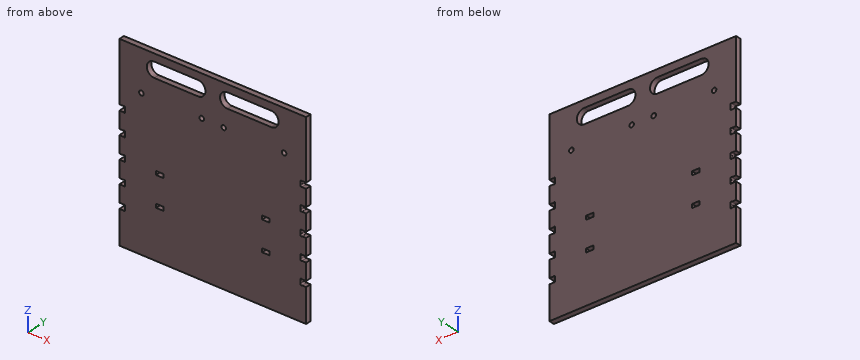
```python
from build123d import *

# Parameters (mm, degrees)
BOSS_EXTRUDE1_DEPTH     = 19.05
SKETCH2_R               = 7.9375
CUT_EXTRUDE1_DEPTH      = 836.260375572
SKETCH3_W               = 25.4
SKETCH3_H               = 12.7
CUT_EXTRUDE2_DEPTH      = 836.260375572
SKETCH4_W               = 444.5
SKETCH4_H               = 114.3
BOSS_EXTRUDE2_DEPTH     = 19.05
CUT_EXTRUDE3_DEPTH      = 836.260375572
CUT_EXTRUDE3_DEPTH_BACK = 836.260375572


with BuildPart() as part:
    # Sketch1 → Boss-Extrude1 (new body)
    with BuildSketch(Plane(origin=(0, 0, 0), x_dir=(1, 0, 0), z_dir=(0, 1, 0))):
        with BuildLine():
            Line((0, 88.9), (0, -114.3))
            Line((0, -114.3), (101.6, -114.3))
            Line((101.6, -114.3), (101.6, 0))
            Line((101.6, 0), (546.1, 0))
            Line((546.1, 0), (546.1, -114.3))
            Line((546.1, -114.3), (647.7, -114.3))
            Line((647.7, -114.3), (647.7, 88.9))
            Line((647.7, 88.9), (633.140128061, 88.9))
            ThreePointArc((633.140128061, 88.9), (628.65, 88.9), (628.65, 93.390128061))
            Line((628.65, 93.390128061), (628.65, 103.459871939))
            ThreePointArc((628.65, 103.459871939), (628.65, 107.95), (633.140128061, 107.95))
            Line((633.140128061, 107.95), (647.7, 107.95))
            Line((647.7, 107.95), (647.7, 165.1))
            Line((647.7, 165.1), (633.140128061, 165.1))
            ThreePointArc((633.140128061, 165.1), (628.65, 165.1), (628.65, 169.590128061))
            Line((628.65, 169.590128061), (628.65, 179.659871939))
            ThreePointArc((628.65, 179.659871939), (628.65, 184.15), (633.140128061, 184.15))
            Line((633.140128061, 184.15), (647.7, 184.15))
            Line((647.7, 184.15), (647.7, 241.3))
            Line((647.7, 241.3), (633.140128061, 241.3))
            ThreePointArc((633.140128061, 241.3), (628.65, 241.3), (628.65, 245.790128061))
            Line((628.65, 245.790128061), (628.65, 255.859871939))
            ThreePointArc((628.65, 255.859871939), (628.65, 260.35), (633.140128061, 260.35))
            Line((633.140128061, 260.35), (647.7, 260.35))
            Line((647.7, 260.35), (647.7, 317.5))
            Line((647.7, 317.5), (633.140128061, 317.5))
            ThreePointArc((633.140128061, 317.5), (628.65, 317.5), (628.65, 321.990128061))
            Line((628.65, 321.990128061), (628.65, 332.059871939))
            ThreePointArc((628.65, 332.059871939), (628.65, 336.55), (633.140128061, 336.55))
            Line((633.140128061, 336.55), (647.7, 336.55))
            Line((647.7, 336.55), (647.7, 393.7))
            Line((647.7, 393.7), (633.140128061, 393.7))
            ThreePointArc((633.140128061, 393.7), (628.65, 393.7), (628.65, 398.190128061))
            Line((628.65, 398.190128061), (628.65, 408.259871939))
            ThreePointArc((628.65, 408.259871939), (628.65, 412.75), (633.140128061, 412.75))
            Line((633.140128061, 412.75), (647.7, 412.75))
            Line((647.7, 412.75), (647.7, 527.05))
            Line((647.7, 527.05), (546.1, 527.05))
            Line((546.1, 527.05), (546.1, 412.75))
            Line((546.1, 412.75), (101.6, 412.75))
            Line((101.6, 412.75), (101.6, 527.05))
            Line((101.6, 527.05), (0, 527.05))
            Line((0, 527.05), (0, 412.75))
            Line((0, 412.75), (14.559871939, 412.75))
            ThreePointArc((14.559871939, 412.75), (19.05, 412.75), (19.05, 408.259871939))
            Line((19.05, 408.259871939), (19.05, 398.190128061))
            ThreePointArc((19.05, 398.190128061), (19.05, 393.7), (14.559871939, 393.7))
            Line((14.559871939, 393.7), (0, 393.7))
            Line((0, 393.7), (0, 336.55))
            Line((0, 336.55), (14.559871939, 336.55))
            ThreePointArc((14.559871939, 336.55), (19.05, 336.55), (19.05, 332.059871939))
            Line((19.05, 332.059871939), (19.05, 321.990128061))
            ThreePointArc((19.05, 321.990128061), (19.05, 317.5), (14.559871939, 317.5))
            Line((14.559871939, 317.5), (0, 317.5))
            Line((0, 317.5), (0, 260.35))
            Line((0, 260.35), (14.559871939, 260.35))
            ThreePointArc((14.559871939, 260.35), (19.05, 260.35), (19.05, 255.859871939))
            Line((19.05, 255.859871939), (19.05, 245.790128061))
            ThreePointArc((19.05, 245.790128061), (19.05, 241.3), (14.559871939, 241.3))
            Line((14.559871939, 241.3), (0, 241.3))
            Line((0, 241.3), (0, 184.15))
            Line((0, 184.15), (14.559871939, 184.15))
            ThreePointArc((14.559871939, 184.15), (19.05, 184.15), (19.05, 179.659871939))
            Line((19.05, 179.659871939), (19.05, 169.590128061))
            ThreePointArc((19.05, 169.590128061), (19.05, 165.1), (14.559871939, 165.1))
            Line((14.559871939, 165.1), (0, 165.1))
            Line((0, 165.1), (0, 107.95))
            Line((0, 107.95), (14.559871939, 107.95))
            ThreePointArc((14.559871939, 107.95), (19.05, 107.95), (19.05, 103.459871939))
            Line((19.05, 103.459871939), (19.05, 93.390128061))
            ThreePointArc((19.05, 93.390128061), (19.05, 88.9), (14.559871939, 88.9))
            Line((14.559871939, 88.9), (0, 88.9))
        make_face()
    extrude(amount=BOSS_EXTRUDE1_DEPTH)

    # Sketch2 → Cut-Extrude1 (cut, through all)
    with BuildSketch(Plane(origin=(0, 19.05, 0), x_dir=(1, 0, 0), z_dir=(0, 1, 0))):
        with Locations(Location((361.95, 25.4, 0), (0, 0, 270))):
            Circle(SKETCH2_R)
        with Locations(Location((285.75, 25.4, 0), (0, 0, 270))):
            Circle(SKETCH2_R)
        with Locations(Location((571.5, 25.4, 0), (0, 0, 270))):
            Circle(SKETCH2_R)
        with Locations(Location((76.2, 25.4, 0), (0, 0, 270))):
            Circle(SKETCH2_R)
    extrude(amount=-CUT_EXTRUDE1_DEPTH, mode=Mode.SUBTRACT)

    # Sketch3 → Cut-Extrude2 (cut, through all)
    with BuildSketch(Plane(origin=(0, 19.05, 0), x_dir=(1, 0, 0), z_dir=(0, 1, 0))):
        with Locations((508, 355.6)):
            Rectangle(SKETCH3_W, SKETCH3_H)
        with Locations((508, 254)):
            Rectangle(SKETCH3_W, SKETCH3_H)
        with Locations((139.7, 254)):
            Rectangle(SKETCH3_W, SKETCH3_H)
        with Locations((139.7, 355.6)):
            Rectangle(SKETCH3_W, SKETCH3_H)
    extrude(amount=-CUT_EXTRUDE2_DEPTH, mode=Mode.SUBTRACT)

    # Sketch4 → Boss-Extrude2 (add)
    with BuildSketch(Plane(origin=(0, 19.05, 0), x_dir=(1, 0, 0), z_dir=(0, 1, 0))):
        with Locations((323.85, -57.15)):
            Rectangle(SKETCH4_W, SKETCH4_H)
        with Locations((323.85, 469.9)):
            Rectangle(SKETCH4_W, SKETCH4_H)
    extrude(amount=-BOSS_EXTRUDE2_DEPTH)

    # Sketch5 → Cut-Extrude3 (cut, two sides: drawn at the far end of the back side and taken through both)
    with BuildSketch(Plane(origin=(0, 19.05, 0), x_dir=(1, 0, 0), z_dir=(0, 1, 0)).offset(-CUT_EXTRUDE3_DEPTH_BACK)):
        with BuildLine():
            Line((374.65, -38.1), (527.05, -38.1))
            ThreePointArc((527.05, -38.1), (552.45, -63.5), (527.05, -88.9))
            Line((527.05, -88.9), (374.65, -88.9))
            ThreePointArc((374.65, -88.9), (349.25, -63.5), (374.65, -38.1))
        make_face()
        with BuildLine():
            Line((273.05, -38.1), (120.65, -38.1))
            ThreePointArc((120.65, -38.1), (95.25, -63.5), (120.65, -88.9))
            Line((120.65, -88.9), (273.05, -88.9))
            ThreePointArc((273.05, -88.9), (298.45, -63.5), (273.05, -38.1))
        make_face()
    extrude(amount=CUT_EXTRUDE3_DEPTH + CUT_EXTRUDE3_DEPTH_BACK, mode=Mode.SUBTRACT)


solid = part.part
```
Source: CAD feature listing. Evaluate the final solid. Frame: model axes, mm. Coordinates: 2 decimals unless noted, no trailing zeros. Loops run counter-clockwise (first coordinate to the right, second up) from the corner with the lowest first, then second, coordinate; pieces in that order, holes last. Notation, with made-up numbers: M -12.5,-6.5 L 9.5,-6.5 A23 cw 9.5,5.5 Z; hole C 33,-31 d9. An arc over 180 degrees is marked long. Use CSV: the item, a comma, the result in double quotes.
(1) Cut plane C-C on x = 203. Return loops of the section in (y, z), and give its area (4 significant figures).
Answers follow:
outline,"M 0,-527.05 L 19.05,-527.05 L 19.05,38.1 L 0,38.1 Z; M 0,88.9 L 19.05,88.9 L 19.05,114.3 L 0,114.3 Z"
area,"11,250 mm²"
(2) Cut plane A-A on z = 63.5. Return loops of the section in (x, y), and give its area (3 significant figures).
Answers follow:
outline,"M 0,0 L 95.25,0 L 95.25,19.05 L 0,19.05 Z; M 298.45,0 L 349.25,0 L 349.25,19.05 L 298.45,19.05 Z; M 552.45,0 L 647.7,0 L 647.7,19.05 L 552.45,19.05 Z"
area,"4,600 mm²"
(3) Cut plane D-D on y = 8. Give the number of separate pieces and of enclosed holes in the cut face, and give its area (3 significant figures).
Answers follow:
separate pieces,"1"
enclosed holes,"10"
area,"390,000 mm²"
(4) Contact query for flat-ended pins moving along their axis: pin 1 (5 mm diameter, centred on y = 9.5, z = -175.5, fed in from -X); pin 2 (6.5 mm diameter, centred on y = 6.5, z = -251.5, fed in from -X); pin 3 (5 mm diameter, centred on y = 13.5, z = -401.5, fed in from +X). Output: stop coordinate, or through.
Answers follow:
pin 1,"x = 19.05"
pin 2,"x = 19.05"
pin 3,"x = 628.65"
(5) Line query: line 1 (X direction, y = 6.75, z = -25.4); line 2 (Z direction, x = 447.5, y = 15.5); line 3 (X direction, y = 13.5, z = -358.5). Output: solid intervals per line, ascending. Write a range as [from, to].
Answers follow:
line 1,"[0, 68.26], [84.14, 277.81], [293.69, 354.01], [369.89, 563.56], [579.44, 647.7]"
line 2,"[-527.05, 38.1], [88.9, 114.3]"
line 3,"[0, 127], [152.4, 495.3], [520.7, 647.7]"
(6) Cut plane B-B on x = 138. Return loops of the section in (y, z), and give its area (3 significant figures).
Answers follow:
outline,"M 0,-527.05 L 19.05,-527.05 L 19.05,-361.95 L 0,-361.95 Z; M 0,-349.25 L 19.05,-349.25 L 19.05,-260.35 L 0,-260.35 Z; M 0,-247.65 L 19.05,-247.65 L 19.05,38.1 L 0,38.1 Z; M 0,88.9 L 19.05,88.9 L 19.05,114.3 L 0,114.3 Z"
area,"10,800 mm²"
